from build123d import *

# Parameters (mm, degrees)
SKETCH1_W           = 37.208239372
SKETCH1_H           = 32.443769696
SKETCH1_R           = 1.52
BOSS_EXTRUDE1_DEPTH = 1.2
SKETCH2_R           = 2.583124011
SKETCH2_R_2         = 2.790118195
SKETCH2_R_3         = 2.5
SKETCH2_R_4         = 2.297434725
SKETCH2_R_5         = 2.229489291
BOSS_EXTRUDE3_DEPTH = 8
SKETCH3_W           = 16.935717079
SKETCH3_H           = 2.186194115
SKETCH3_W_2         = 16.032090178
SKETCH3_H_2         = 2.157044861
SKETCH3_W_3         = 1.807253802
SKETCH3_H_3         = 8.016045089
BOSS_EXTRUDE4_DEPTH = 2


with BuildPart() as part:
    # Sketch1 → Boss-Extrude1 (new body)
    with BuildSketch(Plane(origin=(0, 0, 0), x_dir=(1, 0, 0), z_dir=(0, 1, 0))):
        with Locations((14.595582384, 11.248361917)):
            Rectangle(SKETCH1_W, SKETCH1_H)
        with Locations(Location((0, 0, 0), (0, 0, 270))):
            Circle(SKETCH1_R, mode=Mode.SUBTRACT)
        with Locations(Location((29.24, 0, 0), (0, 0, 270))):
            Circle(SKETCH1_R, mode=Mode.SUBTRACT)
        with Locations(Location((29.24, 23.24, 0), (0, 0, 270))):
            Circle(SKETCH1_R, mode=Mode.SUBTRACT)
        with Locations(Location((0, 23.24, 0), (0, 0, 270))):
            Circle(SKETCH1_R, mode=Mode.SUBTRACT)
    extrude(amount=BOSS_EXTRUDE1_DEPTH)

    # Sketch2 → Boss-Extrude3 (add)
    with BuildSketch(Plane(origin=(0, 1.2, 0), x_dir=(1, 0, 0), z_dir=(0, 1, 0))):
        with Locations(Location((9.028074704, 17.500877086, 0), (0, 0, 270))):
            Circle(SKETCH2_R)
        with Locations(Location((17.6854034, 17.500877086, 0), (0, 0, 270))):
            Circle(SKETCH2_R_2)
        with Locations(Location((8.794880665, 8.493757332, 0), (0, 0, 270))):
            Circle(SKETCH2_R_3)
        with Locations(Location((18.472433282, 8.960145409, 0), (0, 0, 270))):
            Circle(SKETCH2_R_4)
        with Locations(Location((13.604507718, 8.493757332, 0), (0, 0, 270))):
            Circle(SKETCH2_R_5)
    extrude(amount=BOSS_EXTRUDE3_DEPTH)

    # Sketch3 → Boss-Extrude4 (add)
    with BuildSketch(Plane(origin=(0, 1.2, 0), x_dir=(1, 0, 0), z_dir=(0, 1, 0))):
        with Locations((16.184216775, -2.976474459)):
            Rectangle(SKETCH3_W, SKETCH3_H)
        with Locations((13.750253993, 25.225429627)):
            Rectangle(SKETCH3_W_2, SKETCH3_H_2)
        with Locations((-1.115865991, 12.560078386)):
            Rectangle(SKETCH3_W_3, SKETCH3_H_3)
    extrude(amount=BOSS_EXTRUDE4_DEPTH)


solid = part.part
Can you work these out from the model? Positions are in its coordinate system, mm. A direction names the side the tool comes from. Give positions to 0.01 mm unless a question says otherwise; leave off trailing zeros. Write each loop counter-clockwise with the first axis right and the second up, starting at its lowest first coordinate (ties: lowest second). Pieces come first, ordered by that corner, then holes. Notation, with made-up numbers: (-4.5, -11) -> (53.5, -11) arc R16 cw to (53.5, 10) -> close; hole circle Ø8 at (77, 8). An arc over 180 degrees is marked (long way). Answer as a JSON object with one key per item and string values. Group by question number.
Item 1: Suppose I cut it at D-D (y = 6.25). Please give me the cut outline in (x, z), plus the area to 3 significant figures.
Item 2: Suppose I cut it at C-C (z = -23.24). Please give me the cut outline in (x, y).
Item 3: For faces 1 (the face through (-0.212, 2, -13)), 2 (the face through (16, 2, 4.07)), 3 (the face through (7.716, 2, 3)), 4 (the face through (-1, 2, -16.568)), 5 (the face through (8.039, 5.144, -15.115)), which set-ups out of +Z, -Z, +X, -X, +Y, -Y let a thin tool reach every point of the face, with its end or its side?
Item 4: I'm going to push flat-ended pins straight in: P1, Ø0.6, axis at x = 17, y = 2, coming from the +Z side; P2, Ø2.5, axis at x = 12, z = -25.5, coming from the +Y side; P3, Ø1, axis at x = 18, y = 2, coming from the -Z side; P4, Ø1.8, axis at x = 0, z = 0, coming from the +Y side. Where does each tip first touch, or does it pass through?
Item 5: Suppose I cut it at B-B (y = 0.5). Please give me the cut outline in (x, z), plus the area to 3 significant figures.
Item 6: Suppose I cut it at A-A (x = 29.24). Please give me the cut outline in (y, z), plus the area to 3 significant figures.
Item 7: Please list where these lines run through material, in increasing order: line 1 (X direction, y = 0.45, z = -23.24); line 2 (Z direction, x = 18.5, y = 2); line 3 (Y direction, x = 29.5, z = -20.5). Write a range as [from, to].
Item 8: We'd pull the mould along X, two halves only. Please class faces 6 (the face through (33.2, 1, -11)), 7 (the face through (14.962, 5.144, -18.106)), 8 (the face through (27.756, 0.592, -0.33)), 9 (the face through (-4.009, 1, -11)): +X half, -X half, draft (parallel to the pull), parting line (faces both ways), or undercut.
Findings:
{
 "1": {"outline": "circle Ø5 at (8.79, -8.49); circle Ø5.17 at (9.03, -17.5); circle Ø4.46 at (13.6, -8.49); circle Ø5.58 at (17.69, -17.5); circle Ø4.59 at (18.47, -8.96)", "area": "97.3 mm²"},
 "2": {"outline": "(-4.01, 0) -> (-1.52, 0) -> (-1.52, 1.2) -> (-4.01, 1.2) -> close; (1.52, 0) -> (27.72, 0) -> (27.72, 1.2) -> (1.52, 1.2) -> close; (30.76, 0) -> (33.2, 0) -> (33.2, 1.2) -> (30.76, 1.2) -> close"},
 "3": {"face 1": "+Z, -Z, +Y", "face 2": "+Z, +X, -X, +Y", "face 3": "+Z, -X, +Y", "face 4": "-Z, -X, +Y", "face 5": "+Y"},
 "4": {"P1": "stops at z = 4.07", "P2": "stops at y = 3.2", "P3": "stops at z = -26.3", "P4": "passes through"},
 "5": {"outline": "(-4.01, -27.47) -> (33.2, -27.47) -> (33.2, 4.97) -> (-4.01, 4.97) -> close; hole circle Ø3.04 at (0, -23.24); hole circle Ø3.04 at (0, 0); hole circle Ø3.04 at (29.24, -23.24); hole circle Ø3.04 at (29.24, 0)", "area": "1,180 mm²"},
 "6": {"outline": "(0, -27.47) -> (1.2, -27.47) -> (1.2, -24.76) -> (0, -24.76) -> close; (0, -21.72) -> (1.2, -21.72) -> (1.2, -1.52) -> (0, -1.52) -> close; (0, 1.52) -> (1.2, 1.52) -> (1.2, 4.97) -> (0, 4.97) -> close", "area": "31.6 mm²"},
 "7": {"line 1": "x = [-4.01, -1.52], [1.52, 27.72], [30.76, 33.2]", "line 2": "z = [-26.3, -24.15], [-20.17, -14.83], [-11.26, -6.66], [1.88, 4.07]", "line 3": "y = [0, 1.2]"},
 "8": {"face 6": "+X half", "face 7": "undercut", "face 8": "undercut", "face 9": "-X half"}
}
